```python
from build123d import *

# Parameters (mm, degrees)
SKETCH2_W           = 31.6
SKETCH2_H           = 31.6
BOSS_EXTRUDE1_DEPTH = 10
SKETCH13_W          = 4
SKETCH13_H          = 10
BOSS_EXTRUDE2_DEPTH = 12
SKETCH14_R          = 1.75
CUT_EXTRUDE5_DEPTH  = 30
SKETCH9_W           = 25.999998474
SKETCH9_H           = 25.999998474
CUT_EXTRUDE1_DEPTH  = 6
SKETCH10_W          = 16.8
SKETCH10_H          = 23.599998474
CUT_EXTRUDE2_DEPTH  = 2.5
SKETCH11_W          = 9.5
SKETCH11_H          = 9.5
CUT_EXTRUDE3_DEPTH  = 2.5
SKETCH12_R          = 1.1
CUT_EXTRUDE4_DEPTH  = 3
FILLET1_R           = 3
SKETCH15_W          = 17
SKETCH15_H          = 2.800000763
CUT_EXTRUDE6_DEPTH  = 4.5


with BuildPart() as part:
    # Sketch2 → Boss-Extrude1 (new body)
    with BuildSketch(Plane.XY):
        Rectangle(SKETCH2_W, SKETCH2_H)
    extrude(amount=BOSS_EXTRUDE1_DEPTH)

    # Sketch13 → Boss-Extrude2 (add)
    with BuildSketch(Plane.XZ.offset(15.8)):
        with Locations((-9.5, 5)):
            Rectangle(SKETCH13_W, SKETCH13_H)
        with Locations((9.5, 5)):
            Rectangle(SKETCH13_W, SKETCH13_H)
    extrude(amount=BOSS_EXTRUDE2_DEPTH)

    # Sketch14 → Cut-Extrude5 (cut)
    with BuildSketch(Plane.ZY.offset(11.5)):
        with Locations(Location((5, -22.8, 0), (0, 0, 270))):
            Circle(SKETCH14_R)
    extrude(amount=-CUT_EXTRUDE5_DEPTH, mode=Mode.SUBTRACT)

    # Sketch9 → Cut-Extrude1 (cut)
    with BuildSketch(Plane.XY.offset(10)):
        Rectangle(SKETCH9_W, SKETCH9_H)
    extrude(amount=-CUT_EXTRUDE1_DEPTH, mode=Mode.SUBTRACT)

    # Sketch10 → Cut-Extrude2 (cut)
    with BuildSketch(Plane.XY.offset(4)):
        Rectangle(SKETCH10_W, SKETCH10_H)
    extrude(amount=-CUT_EXTRUDE2_DEPTH, mode=Mode.SUBTRACT)

    # Sketch11 → Cut-Extrude3 (cut)
    with BuildSketch(Plane.XY.offset(1.5)):
        with Locations((0, 2.549999952)):
            Rectangle(SKETCH11_W, SKETCH11_H)
    extrude(amount=-CUT_EXTRUDE3_DEPTH, mode=Mode.SUBTRACT)

    # Sketch12 → Cut-Extrude4 (cut)
    with BuildSketch(Plane.XY.offset(4)):
        with Locations((-10.800000191, 2.700000048)):
            Circle(SKETCH12_R)
        with Locations((10.800000191, 2.700000048)):
            Circle(SKETCH12_R)
        with Locations((10.800000191, -9.800000191)):
            Circle(SKETCH12_R)
        with Locations((-10.800000191, -9.800000191)):
            Circle(SKETCH12_R)
    extrude(amount=-CUT_EXTRUDE4_DEPTH, mode=Mode.SUBTRACT)

    # Fillet1
    fillet1_edges = [part.edges().sort_by_distance(p)[0] for p in [
        (0, -15.8, 0),
        (-9.5, -27.8, 0),
        (-9.5, -27.8, 10),
        (13.65, -15.8, 0),
        (9.5, -27.8, 0),
        (9.5, -27.8, 10),
        (0, 15.8, 0),
        (15.8, 0, 0),
        (-13.65, -15.8, 0),
        (-15.8, 0, 0),
        (-15.8, 15.8, 5),
        (15.8, 15.8, 5),
        (15.8, -15.8, 5),
        (-15.8, -15.8, 5),
    ]]
    fillet(fillet1_edges, radius=FILLET1_R)

    # Sketch15 → Cut-Extrude6 (cut)
    with BuildSketch(Plane.XY.offset(10)):
        with Locations((0, 14.399999619)):
            Rectangle(SKETCH15_W, SKETCH15_H)
    extrude(amount=-CUT_EXTRUDE6_DEPTH, mode=Mode.SUBTRACT)


solid = part.part
```
The model under review builds one solid part; all positions refer to its coordinate system, in mm. A direction names the side the tool comes from. Round coordinates to 2 decimals unless told otherwise and drop trailing zeros. Order: outer loops, then holes, each group sorted by start corner. A loop starts at its lowest first (then second) coordinate and runs counter-clockwise, first axis right, second up.
(1) Mouldability with a two-part tool opening along X and no side actions: class faces 6 (the face through (0, 14, 5.5)), 7 (the face through (14.94, -14.9, 6.55)), 8 (the face through (-12.14, -14.94, 0.9)) as released by +X, released by -X, zero draft, split by the parting line, or undercut.
Working result:
face 6: undercut
face 7: released by +X
face 8: zero draft
(2) Take a section at B-B, the plane x = -10.8. State the section outline as (y, z) points.
Working result:
outline: (-27.8, 3) arc R3 ccw to (-24.8, 0) - (12.8, 0) arc R3 ccw to (15.8, 3) - (15.8, 10) - (13, 10) - (13, 4) - (3.8, 4) - (3.8, 1) - (1.6, 1) - (1.6, 4) - (-8.7, 4) - (-8.7, 1) - (-10.9, 1) - (-10.9, 4) - (-13, 4) - (-13, 10) - (-24.8, 10) arc R3 ccw to (-27.8, 7) - close; hole circle Ø3.5 at (-22.8, 5)
(3) Wall thickness on L1, parallel to X at y = -9.8, z = 2.85; L2, parallel to Y at x = -12.5, z = 5.25; L3, parallel to X at y = -26, z = 3: over which ranges is each line inside the solid? List them lowest first.
Working result:
L1: x = -15.8 to -11.9, -9.7 to -8.4, 8.4 to 9.7, 11.9 to 15.8
L2: y = -15.8 to -13, 13 to 15.8
L3: x = -11.5 to -7.5, 7.5 to 11.5
(4) For P1, Ø1.8, axis at x = -11, y = -10.5, coming from the +Z side; P2, Ø2, axis at x = -5.5, z = 6.5, coming from the -Y side; P3, Ø1.4, axis at y = 14.5, z = 8, coming from the -X side, all flat-tipped, find the tip position at first contact; note any pin that passes through.
Working result:
P1: stops at z = 4
P2: stops at y = -15.8
P3: stops at x = -15.63
(5) Take a section at C-C, the plane y = -22.8. State the section outline as (x, z) points.
Working result:
outline: (-11.5, 0) - (-7.5, 0) - (-7.5, 3.25) - (-11.5, 3.25) - close; (-11.5, 6.75) - (-7.5, 6.75) - (-7.5, 10) - (-11.5, 10) - close; (7.5, 0) - (11.5, 0) - (11.5, 3.25) - (7.5, 3.25) - close; (7.5, 6.75) - (11.5, 6.75) - (11.5, 10) - (7.5, 10) - close
(6) Tool access review of faces 1 (the face through (11.39, -8.87, 2.52)), 2 (the face through (12.16, -14.9, 0.86)), 3 (the face through (15.8, 0, 6)), 4 (the face through (0, -2.2, 1)), 5 (the face through (0.18, 14.94, 0.9)): name each direction out of +Z, -Z, +X, -X, +Y, -Y from which nothing blocks a thin tool from reaching the whole face with its end or side.
Working result:
face 1: +Z
face 2: -Z, +X, -Y
face 3: +Z, -Z, +X, +Y, -Y
face 4: +Z, -Z
face 5: -Z, +X, -X, +Y
(7) Take a section at A-A, the plane z = 5. State the section outline as (x, y) points.
Working result:
outline: (-15.8, -12.8) arc R3 ccw to (-12.8, -15.8) - (-11.5, -15.8) - (-11.5, -21.05) - (-7.5, -21.05) - (-7.5, -15.8) - (7.5, -15.8) - (7.5, -21.05) - (11.5, -21.05) - (11.5, -15.8) - (12.8, -15.8) arc R3 ccw to (15.8, -12.8) - (15.8, 12.8) arc R3 ccw to (12.8, 15.8) - (-12.8, 15.8) arc R3 ccw to (-15.8, 12.8) - close; (-11.5, -27.8) - (-7.5, -27.8) - (-7.5, -24.55) - (-11.5, -24.55) - close; (7.5, -27.8) - (11.5, -27.8) - (11.5, -24.55) - (7.5, -24.55) - close; hole (-13, -13) - (13, -13) - (13, 13) - (-13, 13) - close
(8) Take a section at D-D, the plane x = -2. State the section outline as (y, z) points.
Working result:
outline: (-15.8, 3) arc R3 ccw to (-12.8, 0) - (-2.2, 0) - (-2.2, 1.5) - (-11.8, 1.5) - (-11.8, 4) - (-13, 4) - (-13, 10) - (-15.8, 10) - close; (7.3, 0) - (12.8, 0) arc R3 ccw to (15.8, 3) - (15.8, 5.5) - (13, 5.5) - (13, 4) - (11.8, 4) - (11.8, 1.5) - (7.3, 1.5) - close
